Build history of the part. All positions in model axes, mm. Face numbers are marked on the shaded views. A direction names the side the tool comes from. Round coordinates to 2 decimals unless told otherwise and drop trailing zeros. Loops run counter-clockwise (first coordinate to the right, second up) from the corner with the lowest first, then second, coordinate; pieces in that order, holes last.
from build123d import *

# Parameters (mm, degrees)
F1_DEPTH = 25
F3_DEPTH = 37.501
F4_R     = 1
F5_R     = 3
F6_R     = 2


with BuildPart() as f1:
    # F0 (on Top) → F1 (new body)
    with BuildSketch(Plane.XY):
        with BuildLine():
            Line((-69.2244253872, -27.8840622671), (-61.7332391261, -27.8840622671))
            Line((-61.7332391261, -27.8840622671), (-61.7332391261, -23.8840622671))
            Line((-61.7332391261, -23.8840622671), (-65.2244253872, -23.8840622671))
            Line((-65.2244253872, -23.8840622671), (-65.2244253872, 5.6159377329))
            Line((-65.2244253872, 5.6159377329), (-20.2244253872, 5.6159377329))
            Line((-20.2244253872, 5.6159377329), (-20.2244253872, 0.6159377329))
            ThreePointArc((-20.2244253872, 0.6159377329), (-22.9369855286, -2.2909603525), (-20.2244253872, -5.1978584379))
            Line((-20.2244253872, -5.1978584379), (0, 5.6159377329))
            Line((0, 5.6159377329), (80.7755746128, 5.6159377329))
            Line((80.7755746128, 5.6159377329), (80.7755746128, 9.6159377329))
            Line((80.7755746128, 9.6159377329), (-69.2244253872, 9.6159377329))
            Line((-69.2244253872, 9.6159377329), (-69.2244253872, -27.8840622671))
        make_face()
    extrude(amount=F1_DEPTH)

    # F2 (on face) → F3 (cut, through all)
    with BuildSketch(Plane(origin=(0, 9.6159377329, 0), x_dir=(-1, 0, 0), z_dir=(0, 1, 0))):
        Polygon((-68.2755746128, 8.5), (-68.2755746128, 0), (-60.2755746128, 0), (-60.2755746128, 8.5), (-51.2755746128, 8.5), (-51.2755746128, 16.5), (-77.2755746128, 16.5), (-77.2755746128, 8.5), align=None)
    extrude(amount=-F3_DEPTH, mode=Mode.SUBTRACT)

    # F4
    f4_edges = [f1.edges().sort_by_distance(p)[0] for p in [
        (77.275575, 7.615938, 16.5),
        (77.275575, 7.615938, 8.5),
        (51.275575, 7.615938, 16.5),
        (51.275575, 7.615938, 8.5),
        (-65.224425, 5.615938, 12.5),
        (-20.224425, 5.615938, 12.5),
        (-20.224425, 0.615938, 12.5),
        (-65.224425, -23.884062, 12.5),
        (-61.733239, -23.884062, 12.5),
        (-61.733239, -27.884062, 12.5),
        (-69.224425, -27.884062, 12.5),
    ]]
    fillet(f4_edges, radius=F4_R)

    # F5
    f5_edges = [f1.edges().sort_by_distance(p)[0] for p in [
        (80.775575, 7.615938, 0),
        (80.775575, 7.615938, 25),
        (68.275575, 7.615938, 0),
        (60.275575, 7.615938, 0),
        (0, 5.615938, 12.5),
    ]]
    fillet(f5_edges, radius=F5_R)

    # F6
    f6_edges = [f1.edges().sort_by_distance(p)[0] for p in [
        (-69.224425, 9.615938, 12.5),
    ]]
    fillet(f6_edges, radius=F6_R)


solid = f1.part
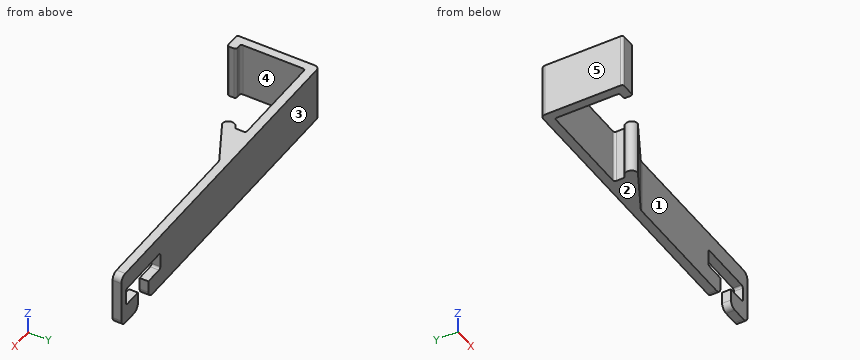
(1) Slice it at B-B on y = 3. List the corners of the cut face in (x, z), plus the area to 3 significant figures.
Responses:
outline: (-69.22, 0) - (-65.22, 0) - (-65.22, 25) - (-69.22, 25) - close; (-20.22, 0) - (-4.89, 0) - (-4.89, 25) - (-20.22, 25) - close
area: 483 mm2
(2) Slice it at C-C on z = 19.75. List the corners of the cut face in (x, y).
Responses:
outline: (-69.22, -26.88) arc R1 ccw to (-68.22, -27.88) - (-62.73, -27.88) arc R1 ccw to (-61.73, -26.88) - (-61.73, -24.88) arc R1 ccw to (-62.73, -23.88) - (-64.22, -23.88) arc R1 cw to (-65.22, -22.88) - (-65.22, 4.62) arc R1 cw to (-64.22, 5.62) - (-21.22, 5.62) arc R1 cw to (-20.22, 4.62) - (-20.22, 1.43) arc R1 cw to (-20.92, 0.48) arc R2.91 ccw to (-20.22, -5.2) - (-0.66, 5.26) arc R3 cw to (0.75, 5.62) - (80.78, 5.62) - (80.78, 9.62) - (-67.22, 9.62) arc R2 ccw to (-69.22, 7.62) - close
(3) Pull direction Y, two halves, no side cores. Call the marked faces 3, 4 and 5: +Y half, -Y half, draft (parallel to the pull), parting line (faces both ways), or undercut.
Responses:
face 3: +Y half
face 4: undercut
face 5: draft
(4) Which spindle directions (+Z, -Z, +X, -X, +Y, -Y) get a long thin tool onto all of the face, cutting with end or side? Do the marked faces 1 and 2. Say none if no direction does.
Responses:
face 1: +Z, -Z, +X, -Y
face 2: -Z, +X, -X, +Y, -Y
(5) Probe line 1 (X direction, y = -10, z = 13); line 2 (X direction, y = -0.5, z = 9.25); line 3 (Y direction, x = 39, z = 14.25). List the from-to ranges inside material, lowest first.
Responses:
line 1: x = -69.22 to -65.22
line 2: x = -69.22 to -65.22, -22.32 to -11.44
line 3: y = 5.62 to 9.62
(6) Slice it at D-D on z = 14. List the corners of the cut face in (x, y).
Responses:
outline: (-69.22, -26.88) arc R1 ccw to (-68.22, -27.88) - (-62.73, -27.88) arc R1 ccw to (-61.73, -26.88) - (-61.73, -24.88) arc R1 ccw to (-62.73, -23.88) - (-64.22, -23.88) arc R1 cw to (-65.22, -22.88) - (-65.22, 4.62) arc R1 cw to (-64.22, 5.62) - (-21.22, 5.62) arc R1 cw to (-20.22, 4.62) - (-20.22, 1.43) arc R1 cw to (-20.92, 0.48) arc R2.91 ccw to (-20.22, -5.2) - (-0.66, 5.26) arc R3 cw to (0.75, 5.62) - (51.28, 5.62) - (51.28, 9.62) - (-67.22, 9.62) arc R2 ccw to (-69.22, 7.62) - close; (77.28, 5.62) - (80.78, 5.62) - (80.78, 9.62) - (77.28, 9.62) - close
(7) Pin check, flat tips, straight feed: P1, Ø12, axis at x = 62, z = 22, coming from the -Y side; P2, Ø6, axis at y = -3, z = 6.5, coming from the +X side; P3, Ø1.2, axis at x = 64, y = 8, coming from the -Z side. Stop position of each tip, or through.
Responses:
P1: stops at y = 5.62
P2: stops at x = -10.5
P3: stops at z = 16.5
(8) Slice it at A-A on z = 7. List the corners of the cut face in (x, y), plus the area to 3 significant figures.
Responses:
outline: (-69.22, -26.88) arc R1 ccw to (-68.22, -27.88) - (-62.73, -27.88) arc R1 ccw to (-61.73, -26.88) - (-61.73, -24.88) arc R1 ccw to (-62.73, -23.88) - (-64.22, -23.88) arc R1 cw to (-65.22, -22.88) - (-65.22, 4.62) arc R1 cw to (-64.22, 5.62) - (-21.22, 5.62) arc R1 cw to (-20.22, 4.62) - (-20.22, 1.43) arc R1 cw to (-20.92, 0.48) arc R2.91 ccw to (-20.22, -5.2) - (-0.66, 5.26) arc R3 cw to (0.75, 5.62) - (60.28, 5.62) - (60.28, 9.62) - (-67.22, 9.62) arc R2 ccw to (-69.22, 7.62) - close; (68.28, 5.62) - (80.78, 5.62) - (80.78, 9.62) - (68.28, 9.62) - close
area: 837 mm2
